Geometry check sheet. Reference: drawing and pictorial views, mm from the part's lowest x, y, z. Give positions to 0.01 mm unless a question says otherwise; leave off trailing zeros. Order: outer loops, then holes, each group sorted by start corner. A loop starts at its lowest first (then second) coordinate and runs counter-clockwise, first axis right, second up. Notation, with made-up numbers: (3, 67) - (8, 67) arc R27 ccw to (8, 91) - close; hole circle Ø11 at (67.25, 6). An arc over 180 degrees is marked (long way). Answer in a Markdown table with one row per item.
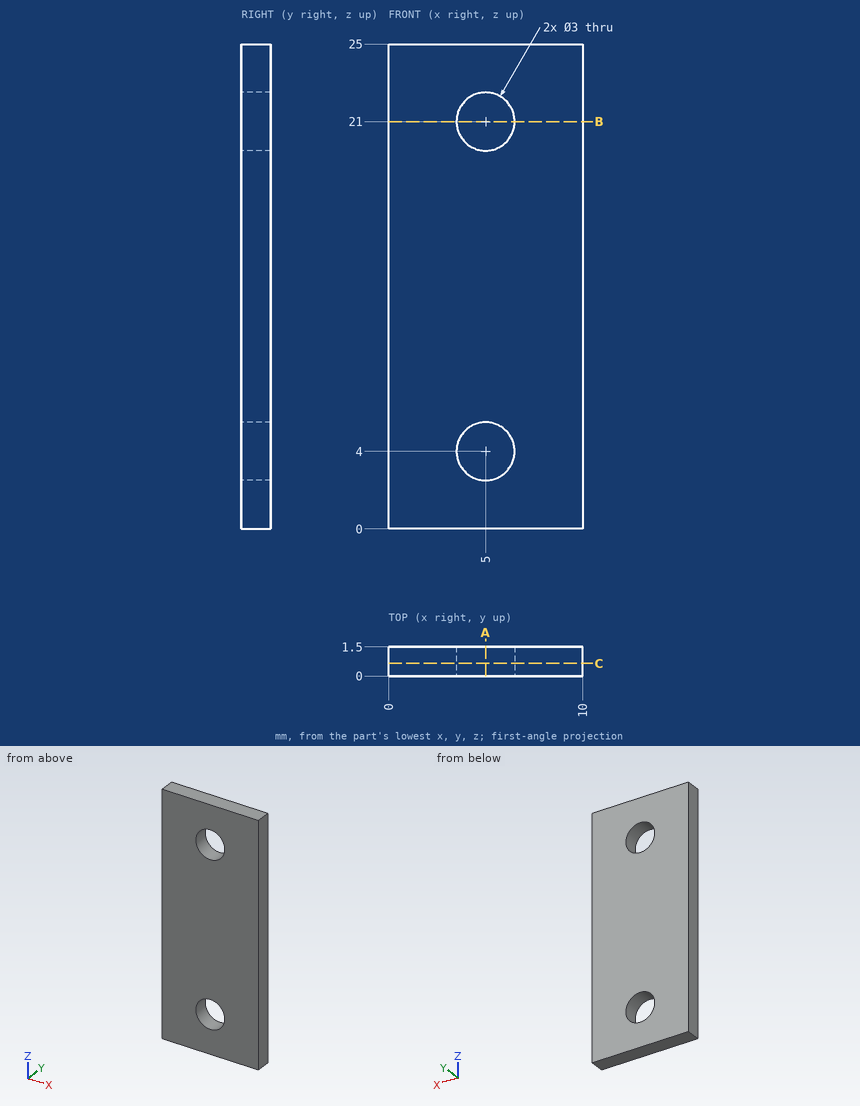
(1) Cross-section at B-B, the plane z = 21. Record the cut outline in (x, y).
Geometry says:
| item | result |
|---|---|
| outline | (0, 0) - (3.5, 0) - (3.5, 1.5) - (0, 1.5) - close; (6.5, 0) - (10, 0) - (10, 1.5) - (6.5, 1.5) - close |
(2) Cross-section at A-A, the plane x = 5. Record the cut outline in (y, z).
Geometry says:
| item | result |
|---|---|
| outline | (0, 0) - (1.5, 0) - (1.5, 2.5) - (0, 2.5) - close; (0, 5.5) - (1.5, 5.5) - (1.5, 19.5) - (0, 19.5) - close; (0, 22.5) - (1.5, 22.5) - (1.5, 25) - (0, 25) - close |
(3) Thickness scan on L1, parallel to Z at x = 5, y = 0.8; L2, parallel to X at y = 0.5, z = 21; L3, parallel to Z at x = 5.75, y = 0.45. Record the ranges inside material, lowest first.
Geometry says:
| item | result |
|---|---|
| L1 | 0 to 2.5, 5.5 to 19.5, 22.5 to 25 |
| L2 | 0 to 3.5, 6.5 to 10 |
| L3 | 0 to 2.7, 5.3 to 19.7, 22.3 to 25 |
(4) Cross-section at C-C, the plane y = 0.65. Record the cut outline in (x, z).
Geometry says:
| item | result |
|---|---|
| outline | (0, 0) - (10, 0) - (10, 25) - (0, 25) - close; hole circle Ø3 at (5, 4); hole circle Ø3 at (5, 21) |
